```python
from build123d import *

# Parameters (mm, degrees)
PAD098_DEPTH    = 3
POCKET028_DEPTH = 3.001
CHAMFER064_SIZE = 1
SKETCH185_R     = 1.6
SKETCH185_W     = 50
SKETCH185_H     = 69.2
POCKET029_DEPTH = 3.001
SKETCH186_R     = 1.6
SKETCH186_W     = 10
SKETCH186_H     = 3
POCKET030_DEPTH = 3.001
POCKET031_DEPTH = 3.001


with BuildPart() as part:
    # Sketch183 → Pad098 (new body)
    with BuildSketch(Plane(origin=(0, 0, 0), x_dir=(-1, 0, 0), z_dir=(0, 1, 0))):
        Polygon((-40, 310), (-30, 310), (-30, 320), (30, 320), (30, 310), (40, 310), (40, 120), (-40, 120), align=None)
    extrude(amount=PAD098_DEPTH)

    # Sketch184 → Pocket028 (cut, through all)
    with BuildSketch(Plane(origin=(0, 0, 0), x_dir=(-1, 0, 0), z_dir=(0, 1, 0))):
        with BuildLine():
            ThreePointArc((-40, 294), (-44, 290), (-40, 286))
            Line((-40, 286), (-35, 286))
            ThreePointArc((-35, 286), (-31, 290), (-35, 294))
            Line((-35, 294), (-40, 294))
        make_face()
        with BuildLine():
            ThreePointArc((-40, 144), (-44, 140), (-40, 136))
            Line((-40, 136), (-35, 136))
            ThreePointArc((-35, 136), (-31, 140), (-35, 144))
            Line((-35, 144), (-40, 144))
        make_face()
        with BuildLine():
            ThreePointArc((40, 136), (44, 140), (40, 144))
            Line((40, 144), (35, 144))
            ThreePointArc((35, 144), (31, 140), (35, 136))
            Line((35, 136), (40, 136))
        make_face()
        with BuildLine():
            ThreePointArc((40, 191), (44, 195), (40, 199))
            Line((40, 199), (35, 199))
            ThreePointArc((35, 199), (31, 195), (35, 191))
            Line((35, 191), (40, 191))
        make_face()
    extrude(amount=POCKET028_DEPTH, mode=Mode.SUBTRACT)

    # Chamfer064
    chamfer064_edges = [part.edges().sort_by_distance(p)[0] for p in [
        (40, 1.5, 310),
        (30, 1.5, 320),
        (40, 1.5, 294),
        (40, 1.5, 286),
        (-40, 1.5, 310),
        (-30, 1.5, 320),
        (40, 1.5, 144),
        (40, 1.5, 136),
        (40, 1.5, 120),
        (-40, 1.5, 120),
        (-40, 1.5, 136),
        (-40, 1.5, 144),
        (-40, 1.5, 191),
        (-40, 1.5, 199),
    ]]
    chamfer(chamfer064_edges, length=CHAMFER064_SIZE)

    # Sketch185 (on Face5 of Chamfer064) → Pocket029 (cut, through all)
    with BuildSketch(Plane(origin=(0, 3, 0), x_dir=(-1, 0, 0), z_dir=(0, 1, 0))):
        with Locations((23.02, 212.62)):
            Circle(SKETCH185_R)
        with Locations((-20.98, 212.62)):
            Circle(SKETCH185_R)
        with Locations((-20.98, 288.7)):
            Circle(SKETCH185_R)
        with Locations((23.02, 288.7)):
            Circle(SKETCH185_R)
        with Locations((1.02, 250.7)):
            Rectangle(SKETCH185_W, SKETCH185_H)
    extrude(amount=-POCKET029_DEPTH, mode=Mode.SUBTRACT)

    # Sketch186 (on Face5 of Pocket029) → Pocket030 (cut, through all)
    with BuildSketch(Plane(origin=(0, 3, 0), x_dir=(-1, 0, 0), z_dir=(0, 1, 0))):
        with Locations((23.62, 163.37)):
            Circle(SKETCH186_R)
        with Locations((3.62, 163.37)):
            Circle(SKETCH186_R)
        with Locations((13.62, 163.37)):
            Rectangle(SKETCH186_W, SKETCH186_H)
    extrude(amount=-POCKET030_DEPTH, mode=Mode.SUBTRACT)

    # Sketch187 → Pocket031 (cut, through all)
    with BuildSketch(Plane.XZ):
        with BuildLine():
            ThreePointArc((-21.019897, 209.69686), (-23.519897, 207.19686), (-21.019897, 204.69686))
            Line((-21.019897, 204.69686), (18.980103, 204.69686))
            ThreePointArc((18.980103, 204.69686), (21.480103, 207.19686), (18.980103, 209.69686))
            Line((18.980103, 209.69686), (-21.019897, 209.69686))
        make_face()
    extrude(amount=-POCKET031_DEPTH, mode=Mode.SUBTRACT)


with BuildPart() as part_1:
    # Body086 placement: moved
    add(part.part.moved(Location((0, 75, 0))))


solid = part_1.part
```
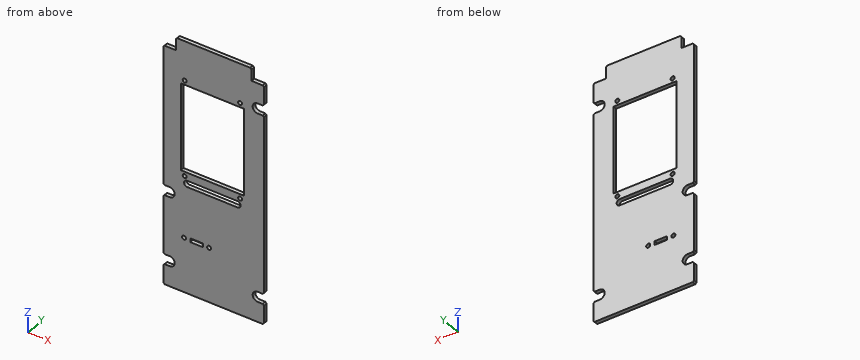
Read the model definition and answer for the solid it produces. Units are mm, in the model's axes. Give positions to 0.01 mm unless a question says otherwise; leave off trailing zeros. Order: outer loops, then holes, each group sorted by start corner. A loop starts at its lowest first (then second) coordinate and runs counter-clockwise, first axis right, second up.
(1) Find section C-C (z = 140). Give the vertices of the cut face in (x, y), plus the area to 3 significant figures.
(2) Straight lines are drawn through the part: L1, parallel to Z at x = 4.5, y = 77.05; L2, parallel to Z at x = 37.5, y = 75.8; L3, parallel to X at y = 77.2, z = 163.37. For each, find the intervals that lie inside material, in ascending order.
(3) Find section A-A (z = 252.5). Give the vertices of the cut face in (x, y).
(4) Given pin 1 (2.5 mm diameter, centred on x = -23.02, z = 288.7, fed in from +Y), flat-ended and moving along its own axis, determine where the tip first touches the part or whether it passes through.
(5) Find section B-B (y = 75.45). Give the number of separate pieces and of enclosed holes in the cut face, plus the area to 3 significant figures.
Result sheet:
1. outline: (-31, 75) - (31, 75) - (31, 78) - (-31, 78) - close
1. area: 186 mm2
2. L1: z = 120 to 204.7, 209.7 to 216.1, 285.3 to 320
2. L2: z = 120 to 136, 144 to 286, 294 to 310
2. L3: x = -40 to -25.22, -22.02 to -18.62, -8.62 to -5.22, -2.02 to 40
3. outline: (-40, 75) - (-26.02, 75) - (-26.02, 78) - (-40, 78) - close; (23.98, 75) - (40, 75) - (40, 78) - (23.98, 78) - close
4. pin 1: passes through
5. separate pieces: 1
5. enclosed holes: 9
5. area: 11,800 mm2
